Here's how the part is built. I have some questions about the finished solid (model axes, mm). Coordinates: 2 decimals unless noted, no trailing zeros. Order: outer loops, then holes, each group sorted by start corner. A loop starts at its lowest first (then second) coordinate and runs counter-clockwise, first axis right, second up. Notation, with made-up numbers: M 85.25,-35 L 140.25,-35 A28 cw 140.25,3 Z; hole C 48.25,40.5 d6. An arc over 180 degrees is marked long. Answer as CSV lines item,"result". Start each with the question number.
```python
from build123d import *

# Parameters (mm, degrees)
SKETCH2_R           = 12.7
BOSS_EXTRUDE1_DEPTH = 558.8
SKETCH3_R           = 44.45
SKETCH3_R_2         = 3.81
BOSS_EXTRUDE2_DEPTH = 6.35
FILLET1_R           = 7.62
FILLET2_R           = 3.175
BOSS_EXTRUDE3_DEPTH = 3.81
FILLET3_R           = 1.27


with BuildPart() as part:
    # Sketch2 → Boss-Extrude1 (new body)
    with BuildSketch(Plane.XY):
        Circle(SKETCH2_R)
    extrude(amount=BOSS_EXTRUDE1_DEPTH)

    # Sketch3 → Boss-Extrude2 (add)
    with BuildSketch(Plane(origin=(0, 0, 0), x_dir=(-1, 0, 0), z_dir=(0, 0, -1))):
        Circle(SKETCH3_R)
        with Locations((0, 31.75)):
            Circle(SKETCH3_R_2, mode=Mode.SUBTRACT)
        with Locations((27.49630657, 15.875)):
            Circle(SKETCH3_R_2, mode=Mode.SUBTRACT)
        with Locations((27.49630657, -15.875)):
            Circle(SKETCH3_R_2, mode=Mode.SUBTRACT)
        with Locations((0, -31.75)):
            Circle(SKETCH3_R_2, mode=Mode.SUBTRACT)
        with Locations((-27.49630657, -15.875)):
            Circle(SKETCH3_R_2, mode=Mode.SUBTRACT)
        with Locations((-27.49630657, 15.875)):
            Circle(SKETCH3_R_2, mode=Mode.SUBTRACT)
    extrude(amount=BOSS_EXTRUDE2_DEPTH)

    # Fillet1
    fillet1_edges = [part.edges().sort_by_distance(p)[0] for p in [
        (-12.7, 0, 0),
    ]]
    fillet(fillet1_edges, radius=FILLET1_R)

    # Fillet2
    fillet2_edges = [part.edges().sort_by_distance(p)[0] for p in [
        (44.45, 0, -6.35),
        (44.45, 0, 0),
    ]]
    fillet(fillet2_edges, radius=FILLET2_R - 0.0001)  # a hair under: the kernel refuses the full size

    # Sketch4 → Boss-Extrude3 (add)
    with BuildSketch(Plane.XY.offset(558.8)):
        with BuildLine():
            Line((-15.750488274, -1.984375), (-22.050683583, 48.021875))
            ThreePointArc((-22.050683583, 48.021875), (0, 73.025), (22.050683583, 48.021875))
            Line((22.050683583, 48.021875), (15.750488274, -1.984375))
            ThreePointArc((15.750488274, -1.984375), (0, -15.875), (-15.750488274, -1.984375))
        make_face()
    extrude(amount=BOSS_EXTRUDE3_DEPTH)

    # Fillet3
    fillet3_edges = [part.edges().sort_by_distance(p)[0] for p in [
        (-12.7, 0, 558.8),
    ]]
    fillet(fillet3_edges, radius=FILLET3_R)


solid = part.part
```
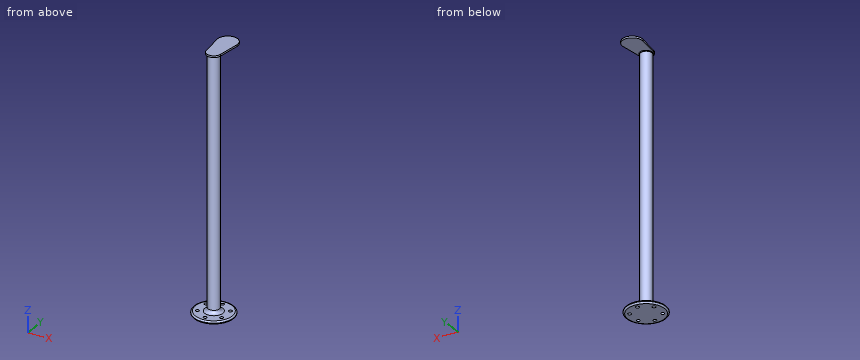
1) Will these pins go through, and if not, where does the flat tip stop? pin 1 Ø9 at (x, y) = (0, -31.75) entering from -Z; pin 2 Ø6 at (y, z) = (17.5, 72.5) entering from -X; pin 3 Ø5 at (x, z) = (12.5, 281) entering from -Y; pin 4 Ø8 at (y, z) = (7, 196.5) entering from +X.
2) Suppose I cut it at A-A on z = 395. Please give me the cut outline in (x, y), plus the area to 3 significant figures.
3) I need wall thicknesses on line 1 (Z direction, x = 3, y = 52); line 2 (X direction, y = 1.5, z = 507.5); line 3 (Z direction, x = 31, y = 14). Which ranges of each line are inside material? Lowest first, please. Write a range as [from, to].
Output:
1,pin 1,"z = -6.35"
1,pin 2,"through"
1,pin 3,"y = -7.83"
1,pin 4,"x = 12.34"
2,outline,"C 0,0 d25.4"
2,area,"507 mm²"
3,line 1,"[558.8, 562.61]"
3,line 2,"[-12.61, 12.61]"
3,line 3,"[-6.35, 0]"
